```python
from build123d import *

# Parameters (mm, degrees)
WYTNIJ_WYCI_GNI_CIE1_START = -5
SZKIC2_W                   = 0.6
SZKIC2_H                   = 0.6
WYTNIJ_WYCI_GNI_CIE1_DEPTH = 3.5
SFAZOWANIE1_SIZE           = 0.75


with BuildPart() as part:
    # Szkic1 → Obrót1 (revolve)
    with BuildSketch(Plane.XY, mode=Mode.PRIVATE) as obr_t1_sk:
        with BuildLine():
            Line((0, 0), (-1.5, 0))
            Line((-1.5, 0), (-1.5, 40))
            Line((-1.5, 40), (-2.8, 40))
            Line((-2.8, 40), (-2.8, 41.5))
            ThreePointArc((-2.8, 41.5), (-1.431782106, 41.948316496), (0, 42.1))
            Line((0, 42.1), (0, 0))
        make_face()
    revolve(obr_t1_sk.sketch.rotate(Axis((0, 0, 0), (0, 1, 0)), 180), axis=Axis((0, 0, 0), (0, 1, 0)))

    # Szkic2 → Wytnij-wyciągnięcie1 (cut)
    with BuildSketch(Plane.XZ.offset(-40).offset(WYTNIJ_WYCI_GNI_CIE1_START)):
        with BuildLine():
            Line((0.3, -0.3), (-0.3, -0.3))
            Line((-0.3, -0.3), (-0.3, -1.469693846))
            ThreePointArc((-0.3, -1.469693846), (0, -1.5), (0.3, -1.469693846))
            Line((0.3, -1.469693846), (0.3, -0.3))
        make_face()
        with BuildLine():
            Line((-0.3, -0.3), (-0.3, 0.3))
            Line((-0.3, 0.3), (-1.469693846, 0.3))
            ThreePointArc((-1.469693846, 0.3), (-1.5, 0), (-1.469693846, -0.3))
            Line((-1.469693846, -0.3), (-0.3, -0.3))
        make_face()
        with BuildLine():
            ThreePointArc((0.3, 1.469693846), (0, 1.5), (-0.3, 1.469693846))
            Line((-0.3, 1.469693846), (-0.3, 0.3))
            Line((-0.3, 0.3), (0.3, 0.3))
            Line((0.3, 0.3), (0.3, 1.469693846))
        make_face()
        with BuildLine():
            ThreePointArc((0.3, 2.783882181), (0.150216331, 2.795967642), (0, 2.8))
            ThreePointArc((0, 2.8), (-0.150216331, 2.795967642), (-0.3, 2.783882181))
            Line((-0.3, 2.783882181), (-0.3, 1.469693846))
            ThreePointArc((-0.3, 1.469693846), (0, 1.5), (0.3, 1.469693846))
            Line((0.3, 1.469693846), (0.3, 2.783882181))
        make_face()
        with BuildLine():
            ThreePointArc((0.3, -1.469693846), (0, -1.5), (-0.3, -1.469693846))
            Line((-0.3, -1.469693846), (-0.3, -2.783882181))
            ThreePointArc((-0.3, -2.783882181), (-0.150216331, -2.795967642), (0, -2.8))
            ThreePointArc((0, -2.8), (0.150216331, -2.795967642), (0.3, -2.783882181))
            Line((0.3, -2.783882181), (0.3, -1.469693846))
        make_face()
        with BuildLine():
            Line((-1.469693846, 0.3), (-2.783882181, 0.3))
            ThreePointArc((-2.783882181, 0.3), (-2.795967642, 0.150216331), (-2.8, 0))
            ThreePointArc((-2.8, 0), (-2.795967642, -0.150216331), (-2.783882181, -0.3))
            Line((-2.783882181, -0.3), (-1.469693846, -0.3))
            ThreePointArc((-1.469693846, -0.3), (-1.5, 0), (-1.469693846, 0.3))
        make_face()
        with BuildLine():
            ThreePointArc((2.8, 0), (2.795967642, 0.150216331), (2.783882181, 0.3))
            Line((2.783882181, 0.3), (1.469693846, 0.3))
            ThreePointArc((1.469693846, 0.3), (1.49240423, 0.150763443), (1.5, 0))
            ThreePointArc((1.5, 0), (1.49240423, -0.150763443), (1.469693846, -0.3))
            Line((1.469693846, -0.3), (2.783882181, -0.3))
            ThreePointArc((2.783882181, -0.3), (2.795967642, -0.150216331), (2.8, 0))
        make_face()
        with BuildLine():
            Line((1.469693846, 0.3), (0.3, 0.3))
            Line((0.3, 0.3), (0.3, -0.3))
            Line((0.3, -0.3), (1.469693846, -0.3))
            ThreePointArc((1.469693846, -0.3), (1.49240423, -0.150763443), (1.5, 0))
            ThreePointArc((1.5, 0), (1.49240423, 0.150763443), (1.469693846, 0.3))
        make_face()
        Rectangle(SZKIC2_W, SZKIC2_H)
    extrude(amount=WYTNIJ_WYCI_GNI_CIE1_DEPTH, mode=Mode.SUBTRACT)

    # Sfazowanie1
    sfazowanie1_edges = [part.edges().sort_by_distance(p)[0] for p in [
        (-1.5, 0, 0),
    ]]
    chamfer(sfazowanie1_edges, length=SFAZOWANIE1_SIZE)


solid = part.part
```
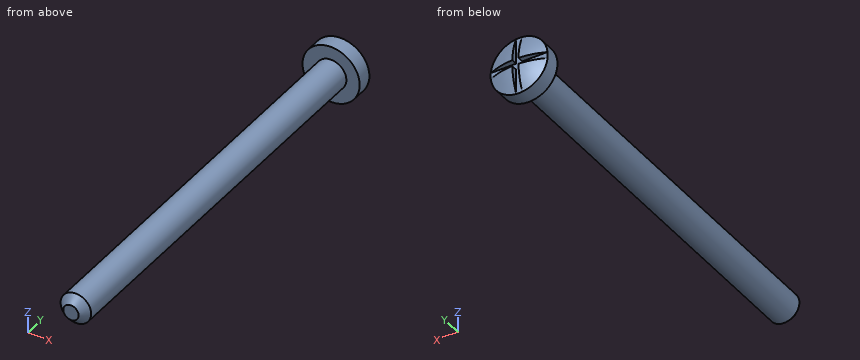
Part model, mm, in its own coordinate system. Coordinates: 2 decimals unless noted, no trailing zeros. Loops run counter-clockwise (first coordinate to the right, second up) from the corner with the lowest first, then second, coordinate; pieces in that order, holes last. Notation, with made-up numbers: (17.25, 58.25) - (65.25, 58.25) arc R13 cw to (65.25, 73.25) - close; hole circle Ø7 at (12.5, 6). An arc over 180 degrees is marked (long way). Write item = value, one per line. Start each with the question number.
Item 1: Cut at A-A, the plane x = 2. Give the cut face in (y, z).
Item 2: Wall check: L1, parallel to Y at x = 0, z = -2.35; L2, parallel to X at y = 3.5, z = 1.3; L3, parallel to Z at x = 0, y = 23. Give the ranges that are in metal, low to high. Write a range as from..to.
Item 3: Flat gauge pins, fed straight in: pin 1 Ø1.5 at (x, z) = (1.5, -1) entering from +Y; pin 2 Ø3 at (y, z) = (7, 0) entering from +X; pin 3 Ø0.6 at (y, z) = (41.5, 1.5) entering from -X. Where does each tip first touch, or does it go through?
The answers:
q1.outline = (40, -1.96) - (41.5, -1.96) arc R6.53 ccw to (41.79, -0.3) - (41.5, -0.3) - (41.5, 0.3) - (41.79, 0.3) arc R6.53 ccw to (41.5, 1.96) - (40, 1.96) - close
q2.L1 = 40..41.5
q2.L2 = -0.75..0.75
q2.L3 = -1.5..1.5
q3.pin_1 = 42.02
q3.pin_2 = 1.5
q3.pin_3 = -2.53
